Input: part model. Units: mm. Frame: model coordinates. A direction names the side the tool comes from. Round coordinates to 2 decimals unless told otherwise and drop trailing zeros. Order: outer loops, then holes, each group sorted by start corner. A loop starts at its lowest first (then second) coordinate and runs counter-clockwise, first axis right, second up. Notation, with made-up numbers: (1.5, -2.75) -> (21.5, -2.75) arc R11 ccw to (21.5, 8.25) -> close; hole circle Ø8 at (60, 19). An arc over 180 degrees is marked (long way). Answer as CSV lines item,"result". Start each with the question number.
1) Line query: L1, parallel to Z at x = 0, y = -10; L2, parallel to X at y = -1, z = 3.5; L3, parallel to X at y = -8, z = 1.5. Output: solid intervals per line, ascending.
2) Section query A-A, the plane z = 0. Output: boundary loops of the cut face in (x, y).
3) Access query for faces 1 (the face through (-0.1, -5.08, -2.7)), 2 (the face through (-2.452, 6.261, 0.772)), 3 (the face through (0, 12.7, 0)). Directions: +Z, -Z, +X, -X, +Y, -Y. A direction counts if a zero-diameter tool reaches every point of the face in a straight line with its end or side. Return the directions, or none.
4) Mould query, pull axis X, two halves, no side actions, for faces 4 (the face through (-15.12, -8.77, -11.59)), 5 (the face through (3.584, -2.576, -4.123)), 6 (the face through (4, 0, 5)). Classes: +X half, -X half, draft (parallel to the pull), parting line (faces both ways), or undercut.
5) Section query B-B, the plane x = 0. Output: boundary loops of the cut face in (y, z), and give its area (3 significant figures).
6) Section query D-D, the plane y = -12.5. Output: boundary loops of the cut face in (x, z).
7) Section query C-C, the plane y = -9. Output: boundary loops of the cut face in (x, z), and give its area (3 significant figures).
8) First-contact query: P1, Ø3, axis at x = 0, z = -4.24, coming from the -Y side; P2, Ø12, axis at x = 13, y = -3.5, coming from the -Z side; P3, Ø1.5, axis at x = -13, z = 13.5, coming from the +Y side; P4, Ø14, axis at x = -3, z = 0.5, coming from the -Y side. Flat tips, straight axial feed; report the tip coordinate or a pass-through.
```python
from build123d import *

# Parameters (mm, degrees)
F0_R      = 19.05
F1_DEPTH  = 17.78
F4_R      = 6.35
F4_R_2    = 2.5388917956
F5_DEPTH  = 12.7
F2_R      = 2.5388917956
F2_R_2    = 2.4229582781
F6_DEPTH  = 7.62
F8_R      = 1.2674888325
F9_DEPTH  = 2.54
F10_DEPTH = 25.4
F11_R     = 2.5702523623
F3_R      = 2.519460743
F12_DEPTH = 12.7


# Not quite as in the source:
# - a feature of the source that left no trace in its solid (it failed there, or was rolled back) is left out


with BuildPart() as f1:
    # F0 (on Front) → F1 (new body)
    with BuildSketch(Plane.XZ):
        Circle(F0_R)
    extrude(amount=F1_DEPTH)

    # F4 (on face) → F5 (cut)
    with BuildSketch(Plane.XZ.offset(17.78)):
        Circle(F4_R)
        Circle(F4_R_2, mode=Mode.SUBTRACT)
    extrude(amount=-F5_DEPTH, mode=Mode.SUBTRACT)

    # F2 (on face) → F6 (cut)
    with BuildSketch(Plane.XZ.offset(17.78)):
        Circle(F2_R)
        Circle(F2_R_2, mode=Mode.SUBTRACT)
        Circle(F2_R_2)
    extrude(amount=-F6_DEPTH, mode=Mode.SUBTRACT)

    # F8 (on face) → F9 (cut)
    with BuildSketch(Plane.XZ.offset(5.08)):
        with Locations((-4.2412145995, 0)):
            Circle(F8_R)
        with Locations((-2.9989916037, 2.9989916037)):
            Circle(F8_R)
        with Locations((0, 4.2412145995)):
            Circle(F8_R)
        with Locations((2.9989916037, 2.9989916037)):
            Circle(F8_R)
        with Locations((4.2412145995, 0)):
            Circle(F8_R)
        with Locations((2.9989916037, -2.9989916037)):
            Circle(F8_R)
        with Locations((0, -4.2412145995)):
            Circle(F8_R)
        with Locations((-2.9989916037, -2.9989916037)):
            Circle(F8_R)
    extrude(amount=-F9_DEPTH, mode=Mode.SUBTRACT)

    # F10 (cut): faces of the model
    f10_faces = [f1.faces().sort_by_distance(p)[0] for p in [
        (-2.9989916037, -2.54, 2.9989916037),
        (-4.2412145995, -2.54, 0),
        (-2.9989916037, -2.54, -2.9989916037),
        (0, -2.54, -4.2412145995),
        (2.9989916037, -2.54, -2.9989916037),
        (4.2412145995, -2.54, 0),
        (2.9989916037, -2.54, 2.9989916037),
        (0, -2.54, 4.2412145995),
    ]]
    extrude(f10_faces, amount=-F10_DEPTH, mode=Mode.SUBTRACT)

    # F11 (on face) + F3 (on face) → F12 (join)
    with BuildSketch(Plane(origin=(0, 0, 0), x_dir=(-1, 0, 0), z_dir=(0, 1, 0))):
        Circle(F11_R)
    with BuildSketch(Plane(origin=(0, 0, 0), x_dir=(-1, 0, 0), z_dir=(0, 1, 0))):
        Circle(F3_R)
    extrude(amount=F12_DEPTH)


solid = f1.part
```
Findings:
1,L1,"z = -19.05 to -6.35, -2.54 to 2.54, 6.35 to 19.05"
1,L2,"x = -18.73 to -4.16, -1.83 to -1.03, 1.03 to 1.83, 4.16 to 18.73"
1,L3,"x = -18.99 to -6.17, -2.05 to 2.05, 6.17 to 18.99"
2,outline,"(-19.05, -17.78) -> (-6.35, -17.78) -> (-6.35, -5.08) -> (-5.51, -5.08) -> (-5.51, 0) -> (-19.05, 0) -> close; (-2.97, -5.08) -> (-2.54, -5.08) -> (-2.54, -10.16) -> (2.54, -10.16) -> (2.54, -5.08) -> (2.97, -5.08) -> (2.97, 0) -> (2.57, 0) -> (2.57, 12.7) -> (-2.57, 12.7) -> (-2.57, 0) -> (-2.97, 0) -> close; (5.51, -5.08) -> (6.35, -5.08) -> (6.35, -17.78) -> (19.05, -17.78) -> (19.05, 0) -> (5.51, 0) -> close"
3,face 1,"-Y"
3,face 2,"+Y"
3,face 3,"+Z, -Z, +X, -X, +Y"
4,face 4,"parting line"
4,face 5,"undercut"
4,face 6,"draft"
5,outline,"(-17.78, -19.05) -> (0, -19.05) -> (0, -5.51) -> (-5.08, -5.51) -> (-5.08, -6.35) -> (-17.78, -6.35) -> close; (-17.78, 6.35) -> (-5.08, 6.35) -> (-5.08, 5.51) -> (0, 5.51) -> (0, 19.05) -> (-17.78, 19.05) -> close; (-10.16, -2.54) -> (-5.08, -2.54) -> (-5.08, -2.97) -> (0, -2.97) -> (0, -2.57) -> (12.7, -2.57) -> (12.7, 2.57) -> (0, 2.57) -> (0, 2.97) -> (-5.08, 2.97) -> (-5.08, 2.54) -> (-10.16, 2.54) -> close"
5,area,"581 mm^2"
6,outline,"circle Ø38.1 at (0, 0); hole circle Ø12.7 at (0, 0)"
7,outline,"circle Ø38.1 at (0, 0); circle Ø5.08 at (0, 0); hole circle Ø12.7 at (0, 0)"
7,area,"1,030 mm^2"
8,P1,"stops at y = -5.08"
8,P2,"stops at z = -17.72"
8,P3,"stops at y = 0"
8,P4,"stops at y = -17.78"
